```python
from build123d import *

# Parameters (mm, degrees)
EXTRUDE_1_DEPTH     = 10
EXTRUDE_2_DEPTH     = 10
CUT_EXTRUDE_1_DEPTH = 57.825808474
CUT_EXTRUDE_2_DEPTH = 57.825808474


with BuildPart() as part:
    # Эскиз2 → Бобышка-Вытянуть1 (new body)
    with BuildSketch(Plane(origin=(0, 0, 0), x_dir=(1, 0, 0), z_dir=(0, 1, 0))):
        Polygon((-44.5, 31.990739153), (44.5, 31.990739153), (44.5, 21.990739153), (18.308398293, -31.990739153), (-44.5, -31.990739153), align=None)
    extrude(amount=EXTRUDE_1_DEPTH)

    # Эскиз3 → Бобышка-Вытянуть2 (add)
    with BuildSketch(Plane.XY.offset(31.990739153)):
        Polygon((-44.5, 0), (0.805588587, 0), (0.805588587, 25), (-4.694411413, 25.017160758), (-44.5, 10), align=None)
    extrude(amount=-EXTRUDE_2_DEPTH)

    # Эскиз4 → Вырез-Вытянуть1 (cut, through all)
    with BuildSketch(Plane(origin=(0, 10, 0), x_dir=(1, 0, 0), z_dir=(0, 1, 0))):
        with BuildLine():
            Line((-40.9, -15.690739153), (-36.1, -15.690739153))
            ThreePointArc((-36.1, -15.690739153), (-35.039339828, -15.251399324), (-34.6, -14.190739153))
            Line((-34.6, -14.190739153), (-34.6, -13.790739153))
            ThreePointArc((-34.6, -13.790739153), (-35.039339828, -12.730078981), (-36.1, -12.290739153))
            Line((-36.1, -12.290739153), (-40.9, -12.290739153))
            ThreePointArc((-40.9, -12.290739153), (-41.960660172, -12.730078981), (-42.4, -13.790739153))
            Line((-42.4, -13.790739153), (-42.4, -14.190739153))
            ThreePointArc((-42.4, -14.190739153), (-41.960660172, -15.251399324), (-40.9, -15.690739153))
        make_face()
        with BuildLine():
            Line((-34.6, 16.609260847), (-34.6, 16.209260847))
            ThreePointArc((-34.6, 16.209260847), (-35.039339828, 15.148600676), (-36.1, 14.709260847))
            Line((-36.1, 14.709260847), (-40.9, 14.709260847))
            ThreePointArc((-40.9, 14.709260847), (-41.960660172, 15.148600676), (-42.4, 16.209260847))
            Line((-42.4, 16.209260847), (-42.4, 16.609260847))
            ThreePointArc((-42.4, 16.609260847), (-41.960660172, 17.669921019), (-40.9, 18.109260847))
            Line((-40.9, 18.109260847), (-36.1, 18.109260847))
            ThreePointArc((-36.1, 18.109260847), (-35.039339828, 17.669921019), (-34.6, 16.609260847))
        make_face()
        with BuildLine():
            Line((-11.3, -14.190739153), (-11.3, -13.790739153))
            ThreePointArc((-11.3, -13.790739153), (-10.860660172, -12.730078981), (-9.8, -12.290739153))
            Line((-9.8, -12.290739153), (-5, -12.290739153))
            ThreePointArc((-5, -12.290739153), (-3.939339828, -12.730078981), (-3.5, -13.790739153))
            Line((-3.5, -13.790739153), (-3.5, -14.190739153))
            ThreePointArc((-3.5, -14.190739153), (-3.939339828, -15.251399324), (-5, -15.690739153))
            Line((-5, -15.690739153), (-9.8, -15.690739153))
            ThreePointArc((-9.8, -15.690739153), (-10.860660172, -15.251399324), (-11.3, -14.190739153))
        make_face()
        with BuildLine():
            Line((-11.3, 16.609260847), (-11.3, 16.209260847))
            ThreePointArc((-11.3, 16.209260847), (-10.860660172, 15.148600676), (-9.8, 14.709260847))
            Line((-9.8, 14.709260847), (-5, 14.709260847))
            ThreePointArc((-5, 14.709260847), (-3.939339828, 15.148600676), (-3.5, 16.209260847))
            Line((-3.5, 16.209260847), (-3.5, 16.609260847))
            ThreePointArc((-3.5, 16.609260847), (-3.939339828, 17.669921019), (-5, 18.109260847))
            Line((-5, 18.109260847), (-9.8, 18.109260847))
            ThreePointArc((-9.8, 18.109260847), (-10.860660172, 17.669921019), (-11.3, 16.609260847))
        make_face()
    extrude(amount=-CUT_EXTRUDE_1_DEPTH, mode=Mode.SUBTRACT)

    # Эскиз5 → Вырез-Вытянуть2 (cut, through all)
    with BuildSketch(Plane(origin=(0, 10, 0), x_dir=(1, 0, 0), z_dir=(0, 1, 0))):
        with BuildLine():
            Line((-19.45, 12.209260847), (-26.45, 12.209260847))
            ThreePointArc((-26.45, 12.209260847), (-33.521067812, 9.280328659), (-36.45, 2.209260847))
            Line((-36.45, 2.209260847), (-36.45, 0.209260847))
            ThreePointArc((-36.45, 0.209260847), (-33.521067812, -6.861806964), (-26.45, -9.790739153))
            Line((-26.45, -9.790739153), (-19.45, -9.790739153))
            ThreePointArc((-19.45, -9.790739153), (-12.378932188, -6.861806964), (-9.45, 0.209260847))
            Line((-9.45, 0.209260847), (-9.45, 2.209260847))
            ThreePointArc((-9.45, 2.209260847), (-12.378932188, 9.280328659), (-19.45, 12.209260847))
        make_face()
    extrude(amount=-CUT_EXTRUDE_2_DEPTH, mode=Mode.SUBTRACT)


solid = part.part
```
CAD build for the part. Positions are in the model's coordinates, mm. A direction names the side the tool comes from. Coordinates: 2 decimals unless noted, no trailing zeros. Order: outer loops, then holes, each group sorted by start corner. A loop starts at its lowest first (then second) coordinate and runs counter-clockwise, first axis right, second up. Notation, with made-up numbers: (35, -20) -> (39, -20) arc R20 cw to (39, -13) -> close; hole circle Ø7 at (2.5, 87). An arc over 180 degrees is marked (long way). Use one line per item in the form item = value. Start each with the question number.
1) Band-saw the part on D-D on z = -27. Give the cut face in (x, y), then the cut area to 3 significant figures.
2) Band-saw the part on C-C on y = 1.5. State how many separate pieces and enclosed holes the cut face has, then the cut area to 3 significant figures.
3) Band-saw the part on A-A on x = -8.5. Give the cut face in (y, z).
4) Tool access for faces 4 (the flat face through (-7, 5, 12.291)), 5 (the flat face through (-1, 5, -31.991)), 6 (the flat face through (-17, 16, 21.991)): list every direction of +Z, -Z, +X, -X, +Y, -Y with a clear straight run to the whole face (end or side of a thin tool).
5) Drop flat-ended pins along their axis: pin 1 (1 mm diameter, centred on y = 2.5, z = -1, fed in from +X); pin 2 (7.5 mm diameter, centred on x = -26, y = 18, fed in from -Z); pin 3 (2 mm diameter, centred on x = 4.5, z = 7, fed in from +Y). Give the stop position or say it passes through.
6) Band-saw the part on B-B on z = 24. Give the cut face in (x, y), then the cut area to 3 significant figures.
7) Drill centre lines: L1, parallel to X at y = 1.5, z = -16.5; L2, parallel to X at y = 4.5, z = 14; L3, parallel to Y at x = 22, z = -6. Where is each one in solid material? Low to high. Write a range as [from, to].
8) Pull direction X, two halves, no side cores. Call faces 1 (the flat face through (-24.319, 17.614, 27.061)), 2 (the flat face through (-13, 10, 31.991)), 3 (the flat face through (-7, 5, -18.109)): +X half, -X half, draft (parallel to the pull), parting line (faces both ways), or undercut.
Entries:
q1.outline = (-44.5, 0) -> (44.5, 0) -> (44.5, 10) -> (-44.5, 10) -> close
q1.area = 890 mm2
q2.separate_pieces = 1
q2.enclosed_holes = 5
q2.area = 4,380 mm2
q3.outline = (0, -31.99) -> (10, -31.99) -> (10, -18.11) -> (0, -18.11) -> close; (0, -14.71) -> (10, -14.71) -> (10, 12.29) -> (0, 12.29) -> close; (0, 15.69) -> (10, 15.69) -> (10, 21.99) -> (23.58, 21.99) -> (23.58, 31.99) -> (0, 31.99) -> close
q4.face_4 = +Y, -Y
q4.face_5 = -Z, +X, -X, +Y, -Y
q4.face_6 = -Z, +X, -X, +Y
q5.pin_1 = 34.56
q5.pin_2 = 21.99
q5.pin_3 = 10
q6.outline = (-44.5, 0) -> (22.19, 0) -> (22.19, 10) -> (0.81, 10) -> (0.81, 25) -> (-4.69, 25.02) -> (-44.5, 10) -> close
q6.area = 1,050 mm2
q7.L1 = [-44.5, -42.4], [-34.6, -11.3], [-3.5, 41.84]
q7.L2 = [-44.5, -42.4], [-34.6, -11.3], [-3.5, 27.04]
q7.L3 = [0, 10]
q8.face_1 = -X half
q8.face_2 = draft
q8.face_3 = undercut
